Verification items for the finished model (mm, model axes). Face numbers are marked on the shaded views. A direction names the side the tool comes from. Coordinates: 2 decimals unless noted, no trailing zeros. Order: outer loops, then holes, each group sorted by start corner. A loop starts at its lowest first (then second) coordinate and runs counter-clockwise, first axis right, second up. Notation, with made-up numbers: (81, 36.25) -> (92, 36.25) arc R15 ccw to (92, 56.25) -> close; hole circle Ø3 at (21.5, 80). An arc over 180 degrees is marked (long way). Write item = value, one per line. Start each with the question number.
from build123d import *

# Parameters (mm, degrees)
SKETCH3_W       = 2
SKETCH3_H       = 1
LPATTERN1_COUNT = 15
LPATTERN1_PITCH = 5


with BuildPart() as part:
    # Sketch2 → Revolve1 (revolve)
    with BuildSketch(Plane(origin=(0, 0, 0), x_dir=(1, 0, 0), z_dir=(0, 1, 0))):
        Polygon((0, 0), (10, 0), (10, 3), (6, 3), (6, 6), (10, 6), (10, 9), (5, 9), (5, 200), (0, 200), align=None)
    revolve(axis=Axis((0, 0, 0), (0, 0, -1)))

    # Sketch3 → Cut-Revolve1 (revolve, cut)
    with BuildSketch(Plane(origin=(0, 0, 0), x_dir=(1, 0, 0), z_dir=(0, 1, 0))):
        with Locations((4, 195.5)):
            Rectangle(SKETCH3_W, SKETCH3_H)
    cut_revolve1 = revolve(axis=Axis((0, 0, 0), (0, 0, -1)), mode=Mode.SUBTRACT)

    # LPattern1: Cut-Revolve1 ×15
    with Locations(*[(0, 0, i * LPATTERN1_PITCH) for i in range(1, LPATTERN1_COUNT)]):
        add(cut_revolve1, mode=Mode.SUBTRACT)


solid = part.part
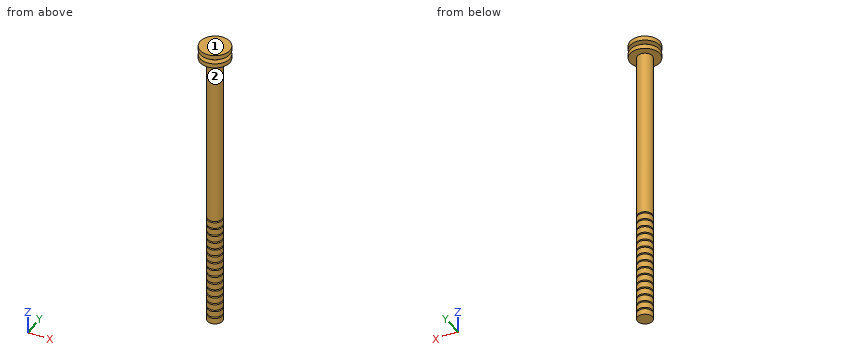
Item 1: Tool access check on the marked faces 1 and 2. Record the directions out of +Z, -Z, +X, -X, +Y, -Y that give a thin tool (end or side, any length) a straight path to the whole face; none if there is none.
Item 2: Gauge pin test, flat ends, axial feed: P1, Ø12, axis at y = -3, z = -115.5, coming from the +X side; P2, Ø1, axis at x = -4, y = 4.5, coming from the -Z side; P3, Ø1.5, axis at y = 7.5, z = -98.5, coming from the +X side. Record the tip position at first contact, or that the pin passes through.
Item 3: Thickness scan on line 1 (Z direction, x = -8.5, y = 3.25); line 2 (Y direction, x = -1, z = -185.5); line 3 (Z direction, x = 3.25, y = -4). Record the ranges inside material, lowest first.
Item 4: Section check A-A (z = -82). Record the boundary of the cut face in (x, y), then the cut area to 3 significant figures.
Filled sheet:
q1.face_1 = +Z, +X, -X, +Y, -Y
q1.face_2 = -Z
q2.P1 = 5
q2.P2 = -9
q2.P3 = through
q3.line_1 = -9 to -6, -3 to 0
q3.line_2 = -2.83 to 2.83
q3.line_3 = -9 to 0
q4.outline = circle Ø10 at (0, 0)
q4.area = 78.5 mm^2
